Autodesk Inventor part; units mm, degrees
ref_plane "YZ Plane" through (0, 0, 0) normal (1, 0, 0) x (0, 1, 0)
ref_plane "XZ Plane" through (0, 0, 0) normal (0, 1, 0) x (-1, 0, 0)
sketch "Sketch1" plane through (0, 0, 0) normal (0, 1, 0) x (-1, 0, 0)
  line L0 (-12, 14) -> (12, 14) construction
  line L1 (14, 12) -> (14, -12) construction
  line L2 (12, -14) -> (-12, -14) construction
  line L3 (-14, -12) -> (-14, 12) construction
  line L4 (-14, 14) -> (14, -14) construction
  line L5 (14, 14) -> (-14, -14) construction
  arc A0 (14, 12) -> (12, 14) centre (12, 12) ccw construction
  arc A1 (12, -14) -> (14, -12) centre (12, -12) ccw construction
  arc A2 (-14, -12) -> (-12, -14) centre (-12, -12) ccw construction
  arc A3 (-12, 14) -> (-14, 12) centre (-12, 12) ccw construction
  line L6 (-12, -15) -> (12, -15)
  arc A4 (12, -15) -> (15, -12) centre (12, -12) ccw
  line L7 (15, -12) -> (15, 12)
  arc A5 (15, 12) -> (12, 15) centre (12, 12) ccw
  line L8 (12, 15) -> (-12, 15)
  arc A6 (-12, 15) -> (-15, 12) centre (-12, 12) ccw
  line L9 (-15, 12) -> (-15, -12)
  arc A7 (-15, -12) -> (-12, -15) centre (-12, -12) ccw
  line L10 (13, -12) -> (13, 12)
  arc A8 (13, 12) -> (12, 13) centre (12, 12) ccw
  line L11 (12, 13) -> (-12, 13)
  arc A9 (-12, 13) -> (-13, 12) centre (-12, 12) ccw
  line L12 (-13, 12) -> (-13, -12)
  arc A10 (-13, -12) -> (-12, -13) centre (-12, -12) ccw
  line L13 (-12, -13) -> (12, -13)
  arc A11 (12, -13) -> (13, -12) centre (12, -12) ccw
  point P0 (0, 0)
  point P1 (0, 0)
  point P2 (0, 0)
  dimension "d10" = 2
  dimension "depth" = 30
  dimension "width" = 30
  dimension "thickness" = 2
sketch "Sketch3" plane through (0, 0, 0) normal (1, 0, 0) x (0, 1, 0)
  line L0 (0, 0) -> (200, 0)
  line L1 (200, 0) -> (200, 1000) construction
  line L2 (200, 1000) -> (0, 1000)
  arc A0 (200, 0) -> (200, 1000) centre (200, 500) ccw
  dimension "d29" = 200
  dimension "d30" = 1000
  dimension "d31" = 500
sweep "Sweep1" add profiles "Sketch1" path "Sketch3"
sketch "Sketch4" plane through (-15, 0, 12) normal (-1, 0, 0) x (0, 0, 1)
  line L0 (-24, 0) -> (0, 0)
  line L1 (-12, 0) -> (-12, 351.1006) construction
  line L2 (1000, 0) -> (976, 0)
  line L3 (988, 0) -> (988, 177.1323) construction
  point P0 (-12, 50)
  point P1 (-12, 100)
  point P2 (988, 50)
  point P3 (988, 100)
  dimension "d34" = 50
  dimension "d35" = 50
  dimension "d36" = 50
  dimension "d37" = 50
hole "Hole2" at (-15, 50, 0) at (-15, 100, 0) at (-15, 50, 1000) at (-15, 100, 1000) direction (1, 0, 0) diameter 9 depth 20.2 tip angle 118
ref_plane "Work Plane1" through (12, 200, 1000) normal (0, 0, -1) x (-1, 0, 0)
ref_plane "Work Plane2" through (0, 715, 500) normal (0, -1, 0) x (1, 0, 0)
equation "\"d10\" = thickness"
equation "\"d31\" = 0.5 * d30"
properties part number "Luk R1000" material "Steel"
Read the model definition and answer for the solid it produces. Units are mm, in the model's axes. A direction names the side the tool comes from. Coordinates: 2 decimals unless noted, no trailing zeros. Loops run counter-clockwise (first coordinate to the right, second up) from the corner with the lowest first, then second, coordinate; pieces in that order, holes last. Notation, with made-up numbers: (26.25, 89) -> (49.25, 89) arc R14 ccw to (49.25, 109) -> close; hole circle Ø6 at (-39, 59). An arc over 180 degrees is marked (long way). Return JSON: item names as keys, results as strings.
Item 1: For faces 1 (the flat face through (0, 99, 985)), 2 (the flat face through (0, 99, 1013)), 3 (the flat face through (13, 700, 536)), determine the directions among +Z, -Z, +X, -X, +Y, -Y from which every point of the face is accessible in a straight line to the end or side of a thin tool.
Answers:
{"face 1": "+X, -X, -Y", "face 2": "-Y", "face 3": "none"}
Item 2: Find section A-A (y = 149). Count the separate pieces of the cut face and the enclosed holes in it, plus the area to 3 significant figures.
Answers:
{"separate pieces": "2", "enclosed holes": "2", "area": "434 mm2"}
Item 3: Flat-ended cylindrical pins translate along their axes: P1, Ø4, axis at x = -7.5, y = 403.5, coming from the +Z side; P2, Ø1, axis at x = 0, z = 714.5, coming from the -Y side; P3, Ø7, axis at y = 100, z = 0, coming from the -X side. Find the tip coordinate at first contact, or state that the pin passes through.
Answers:
{"P1": "stops at z = 973.94", "P2": "stops at y = 634.74", "P3": "stops at x = 13"}
Item 4: Find section B-B (z = 500). Determine the outline of the cut face in (x, y), plus the area to 3 significant figures.
Answers:
{"outline": "(-15, 688) arc R3 ccw to (-12, 685) -> (12, 685) arc R3 ccw to (15, 688) -> (15, 712) arc R3 ccw to (12, 715) -> (-12, 715) arc R3 ccw to (-15, 712) -> close; hole (-13, 688) arc R1 ccw to (-12, 687) -> (12, 687) arc R1 ccw to (13, 688) -> (13, 712) arc R1 ccw to (12, 713) -> (-12, 713) arc R1 ccw to (-13, 712) -> close", "area": "217 mm2"}
Item 5: Find section C-C (x = -5). Determine the outline of the cut face in (y, z), plus the area to 3 significant figures.
Answers:
{"outline": "(0, -15) -> (200, -15) arc R515 ccw to (200, 1015) -> (0, 1015) -> (0, 1013) -> (200, 1013) arc R513 cw to (200, -13) -> (0, -13) -> close; (0, 13) -> (200, 13) arc R487 ccw to (200, 987) -> (0, 987) -> (0, 985) -> (200, 985) arc R485 cw to (200, 15) -> (0, 15) -> close", "area": "7,880 mm2"}
Item 6: Find the intervals of material crossed by probe 1 along Z at (x, y) = (9.5, 81); probe 2 along Z at (x, y) = (4, 458); probe 3 along X at (y, z) = (618, 781.5), in increasing order.
Answers:
{"probe 1": "z = -15 to -13, 13 to 15, 985 to 987, 1013 to 1015", "probe 2": "z = 54.29 to 56.6, 86.96 to 89.32, 910.68 to 913.04, 943.4 to 945.71", "probe 3": "x = -15 to -13, 13 to 15"}
Item 7: For a pull along Y with two mould halves and no side action, classify faces 4 (the cylindrical face through (-0.168, 686.882, 510.709)), 5 (the flat face through (0, 101, 15)), 6 (the cylindrical face through (-0.168, 714.875, 511.325)) as +Y half, -Y half, draft (parallel to the pull), parting line (faces both ways), or undercut.
Answers:
{"face 4": "undercut", "face 5": "draft", "face 6": "+Y half"}
